The listing builds one solid part. Answer for the finished solid, in the listing's coordinates (mm). Face numbers are marked on the shaded views. A direction names the side the tool comes from. Give positions to 0.01 mm unless a question says otherwise; leave off trailing zeros. Loops run counter-clockwise (first coordinate to the right, second up) from the corner with the lowest first, then second, coordinate; pieces in that order, holes last. Notation, with made-up numbers: (22.25, 72) - (68.25, 72) arc R7 cw to (68.25, 80) - close; hole circle Ø11 at (8.25, -5). An arc over 180 degrees is marked (long way). Answer as CSV lines item,"result". Start each with the question number.
1) A cutting plane is placed at B-B (x = -6.7). Determine the outline of the cut face in (y, z), and give its area (3 significant figures).
2) Flat-ended cylindrical pins translate along their axes: pin 1 (4 mm diameter, centred on x = -8.5, y = 7.5, fed in from +Z); pin 2 (5 mm diameter, centred on y = 15.9, z = 21.21, fed in from -X); pin 3 (11 mm diameter, centred on x = -4.5, y = 33, fed in from +Z). Find the tip coordinate at first contact, or state that the pin passes through.
3) For a pull along X with two mould halves and no side action, classify the marked faces 3, 4 and 5 as pulls with the +X half, pulls with the -X half, needs draft (parallel to the pull), parting line crosses it, or undercut.
4) For the marked faces 1 and 2, determine the directions among +Z, -Z, +X, -X, +Y, -Y from which every point of the face is accessible in a straight line to the end or side of a thin tool.
5) A cutting plane is placed at A-A (x = 18). Determine the outline of the cut face in (y, z).
6) Find the intervals of material crossed by line 1 along Y through (x, z) = (47.55, 3.4); line 2 along X through (y, z) = (53, 36); line 3 along X through (y, z) = (58, 27), in increasing order.
7) A cutting plane is placed at C-C (x = -34). Determine the outline of the cut face in (y, z).
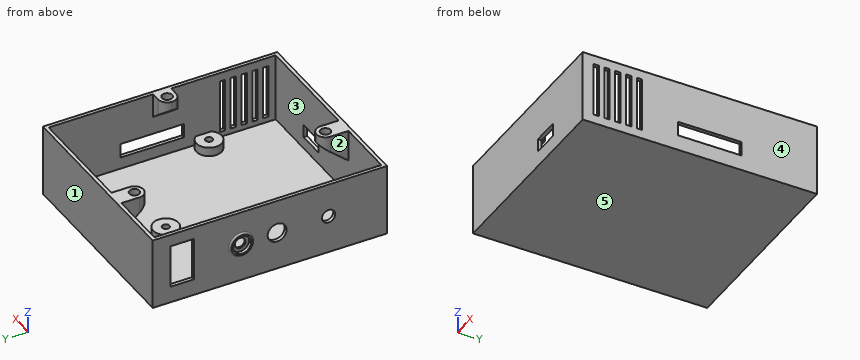
```python
from build123d import *

# Parameters (mm, degrees)
SKETCH1_W                = 110
SKETCH1_H                = 130
BOSS_EXTRUDE1_DEPTH      = 40
SHELL1_T                 = -2
SKETCH2_W                = 15
SKETCH2_H                = 7.298661228
CUT_EXTRUDE1_DEPTH       = 2
SKETCH3_W                = 8
SKETCH3_H                = 35
CUT_EXTRUDE2_DEPTH       = 2
SKETCH5_R                = 3
SKETCH5_R_2              = 5.25
SKETCH5_R_3              = 3.7
SKETCH5_W                = 24
SKETCH5_H                = 13
CUT_EXTRUDE3_DEPTH       = 2
SKETCH6_W                = 30
SKETCH6_H                = 3
CUT_EXTRUDE4_DEPTH       = 2
SKETCH7_R                = 7
SKETCH7_R_2              = 2
BOSS_EXTRUDE2_DEPTH      = 5
BOSS_EXTRUDE3_DEPTH      = 5
FILLET1_R                = 5
BOSS_EXTRUDE4_DEPTH      = 5
BOSS_EXTRUDE4_DEPTH_BACK = 5
FILLET2_R                = 5
CUT_EXTRUDE9_REACH       = 96.074
SKETCH11_R               = 2.8
CUT_EXTRUDE10_REACH      = 96.074
SKETCH13_R               = 2.85
FILLET1_OF_MIRROR1_R     = 5
SKETCH14_R               = 5
CUT_EXTRUDE11_DEPTH      = 1
BOSS_EXTRUDE5_START      = 1
SKETCH15_R               = 6
SKETCH15_R_2             = 5
BOSS_EXTRUDE5_DEPTH      = 1
FILLET3_R                = 1


with BuildPart() as part:
    # Sketch1 → Boss-Extrude1 (new body)
    with BuildSketch(Plane.XY):
        Rectangle(SKETCH1_W, SKETCH1_H)
    extrude(amount=BOSS_EXTRUDE1_DEPTH)

    # Shell1
    shell1_openings = [part.faces().sort_by_distance(p)[0] for p in [
        (0, 0, 40),
    ]]
    offset(amount=SHELL1_T, openings=shell1_openings, kind=Kind.INTERSECTION)

    # Sketch2 → Cut-Extrude1 (cut)
    with BuildSketch(Plane.XZ.offset(65)):
        with Locations((17.5, 12.249330614)):
            Rectangle(SKETCH2_W, SKETCH2_H)
    extrude(amount=-CUT_EXTRUDE1_DEPTH, mode=Mode.SUBTRACT)

    # Sketch3 → Cut-Extrude2 (cut)
    with BuildSketch(Plane(origin=(55, 0, 0), x_dir=(0, 0, -1), z_dir=(1, 0, 0))):
        with Locations((-12.6, 5.5)):
            Rectangle(SKETCH3_W, SKETCH3_H)
    extrude(amount=-CUT_EXTRUDE2_DEPTH, mode=Mode.SUBTRACT)

    # Sketch5 → Cut-Extrude3 (cut)
    with BuildSketch(Plane.ZY.offset(55)):
        with Locations((21.210132709, 15.904045732)):
            Circle(SKETCH5_R)
        with Locations((21.210132709, -4.045954268)):
            Circle(SKETCH5_R_2)
        with Locations((21.210132709, -32.595954268)):
            Circle(SKETCH5_R_3)
        with Locations((21.210132709, 48.5)):
            Rectangle(SKETCH5_W, SKETCH5_H)
    extrude(amount=-CUT_EXTRUDE3_DEPTH, mode=Mode.SUBTRACT)

    # Sketch6 → Cut-Extrude4 (cut)
    with BuildSketch(Plane(origin=(55, 0, 0), x_dir=(0, 0, -1), z_dir=(1, 0, 0))):
        with Locations((-20, -33.5)):
            Rectangle(SKETCH6_W, SKETCH6_H)
        with Locations((-20, -39.5)):
            Rectangle(SKETCH6_W, SKETCH6_H)
        with Locations((-20, -45.5)):
            Rectangle(SKETCH6_W, SKETCH6_H)
        with Locations((-20, -51.5)):
            Rectangle(SKETCH6_W, SKETCH6_H)
        with Locations((-20, -57.5)):
            Rectangle(SKETCH6_W, SKETCH6_H)
    extrude(amount=-CUT_EXTRUDE4_DEPTH, mode=Mode.SUBTRACT)

    # Sketch7 → Boss-Extrude2 (add)
    # profile 1 of 2: a face of its own
    with BuildSketch(Plane.XY.offset(2)):
        with Locations((-6.7, 30.999839281)):
            Circle(SKETCH7_R)
        with Locations((-6.7, 30.999839281)):
            Circle(SKETCH7_R_2, mode=Mode.SUBTRACT)
    # profile 2 of 2: a face of its own
    with BuildSketch(Plane.XY.offset(2)):
        with Locations((47.55, -23.000160719)):
            Circle(SKETCH7_R)
        with Locations((47.55, -23.000160719)):
            Circle(SKETCH7_R_2, mode=Mode.SUBTRACT)
    extrude(amount=BOSS_EXTRUDE2_DEPTH)

    # Sketch9 → Boss-Extrude3 (add, symmetric)
    with BuildSketch(Plane(origin=(-15, 0, 0), x_dir=(0, 0, -1), z_dir=(1, 0, 0))):
        Polygon((-40, 63), (-40, 48), (-35, 48), (-22.413505532, 63), align=None)
    boss_extrude3 = extrude(amount=BOSS_EXTRUDE3_DEPTH, both=True)

    # Fillet1
    fillet1_edges = [part.edges().sort_by_distance(p)[0] for p in [
        (-10, 48, 37.5),
        (-20, 48, 37.5),
    ]]
    fillet(fillet1_edges, radius=FILLET1_R - 0.0001)  # a hair under: the kernel refuses the full size

    # Sketch10 → Boss-Extrude4 (add, two sides: drawn at the far end of the back side and taken through both)
    with BuildSketch(Plane(origin=(0, 0, 0), x_dir=(1, 0, 0), z_dir=(0, 1, 0)).offset(-BOSS_EXTRUDE4_DEPTH_BACK)):
        Polygon((53, -26.609003688), (53, -40), (43, -40), (43, -35), align=None)
    extrude(amount=BOSS_EXTRUDE4_DEPTH + BOSS_EXTRUDE4_DEPTH_BACK)

    # Fillet2
    fillet2_edges = [part.edges().sort_by_distance(p)[0] for p in [
        (43, 5, 37.5),
        (43, -5, 37.5),
    ]]
    fillet(fillet2_edges, radius=FILLET2_R - 0.0001)  # a hair under: the kernel refuses the full size

    # Cut-Extrude9: up to this plane
    cut_extrude9_end = Plane(origin=(-20, 48, 35), z_dir=(0, -0.6427876096865434, -0.7660444431189748))
    # Sketch11 → Cut-Extrude9 (cut, up to the surface)
    with BuildSketch(Plane.XY.offset(40), mode=Mode.PRIVATE) as cut_extrude9_sk1:
        with Locations((-15, 53)):
            Circle(SKETCH11_R)
    cut_extrude9_tool1 = split(extrude(cut_extrude9_sk1.sketch, amount=-CUT_EXTRUDE9_REACH, mode=Mode.PRIVATE), bisect_by=cut_extrude9_end, keep=Keep.BOTH, mode=Mode.PRIVATE)
    cut_extrude9 = cut_extrude9_tool1.solids().sort_by_distance((-15, 53, 40))[0]
    add(cut_extrude9, mode=Mode.SUBTRACT)

    # Cut-Extrude10: up to this plane
    cut_extrude10_end = Plane(origin=(43, -5, 35), z_dir=(-0.6427876096865458, 0, -0.7660444431189727))
    # Sketch13 → Cut-Extrude10 (cut, up to the surface)
    with BuildSketch(Plane.XY.offset(40), mode=Mode.PRIVATE) as cut_extrude10_sk1:
        with Locations((48, 0)):
            Circle(SKETCH13_R)
    cut_extrude10_tool1 = split(extrude(cut_extrude10_sk1.sketch, amount=-CUT_EXTRUDE10_REACH, mode=Mode.PRIVATE), bisect_by=cut_extrude10_end, keep=Keep.BOTH, mode=Mode.PRIVATE)
    add(cut_extrude10_tool1.solids().sort_by_distance((48, 0, 40))[0], mode=Mode.SUBTRACT)

    # Mirror1: Boss-Extrude3, Cut-Extrude9 across plane
    add(boss_extrude3.mirror(Plane.ZX))
    add(cut_extrude9.mirror(Plane.ZX), mode=Mode.SUBTRACT)

    # Fillet1 of Mirror1
    fillet1_of_mirror1_edges = [part.edges().sort_by_distance(p)[0] for p in [
        (-10, -48, 37.5),
        (-20, -48, 37.5),
    ]]
    fillet(fillet1_of_mirror1_edges, radius=FILLET1_OF_MIRROR1_R - 0.0001)  # a hair under: the kernel refuses the full size

    # Sketch14 → Cut-Extrude11 (cut)
    with BuildSketch(Plane.ZY.offset(55)):
        with Locations((21.210132709, 15.904045732)):
            Circle(SKETCH14_R)
    extrude(amount=-CUT_EXTRUDE11_DEPTH, mode=Mode.SUBTRACT)

    # Sketch15 → Boss-Extrude5 (add)
    with BuildSketch(Plane.ZY.offset(55).offset(BOSS_EXTRUDE5_START)):
        with Locations(Location((21.210132709, 15.904045732, 0), (0, 0, 180))):
            Circle(SKETCH15_R)
        with Locations((21.210132709, 15.904045732)):
            Circle(SKETCH15_R_2, mode=Mode.SUBTRACT)
    extrude(amount=-BOSS_EXTRUDE5_DEPTH)

    # Fillet3
    fillet3_edges = [part.edges().sort_by_distance(p)[0] for p in [
        (-55, 15.904045732, 27.210132709),
    ]]
    fillet(fillet3_edges, radius=FILLET3_R - 0.0001)  # a hair under: the kernel refuses the full size


solid = part.part
```
Ans:
1,outline,"(-65, 0) - (65, 0) - (65, 40) - (63, 40) - (63, 2) - (38, 2) - (38, 7) - (33, 7) - (33, 2) - (29, 2) - (29, 7) - (24, 7) - (24, 2) - (-63, 2) - (-63, 40) - (-65, 40) - close"
1,area,"462 mm2"
2,pin 1,"z = 2"
2,pin 2,"x = 53"
2,pin 3,"z = 7"
3,face 3,"undercut"
3,face 4,"pulls with the +X half"
3,face 5,"needs draft"
4,face 1,"+Z, -Z, +X, -X, +Y"
4,face 2,"+Z"
5,outline,"(-65, 0) - (65, 0) - (65, 40) - (63, 40) - (63, 2) - (-63, 2) - (-63, 8.6) - (-65, 8.6) - close; (-65, 15.9) - (-63, 15.9) - (-63, 40) - (-65, 40) - close"
6,line 1,"-65 to -63, -30 to -25, -21 to -16, 63 to 65"
6,line 2,"-55 to -53, -20 to -17.8, -12.2 to -10, 53 to 55"
6,line 3,"-55 to -53, -20 to -10, 53 to 55"
7,outline,"(-65, 0) - (65, 0) - (65, 40) - (63, 40) - (63, 2) - (-63, 2) - (-63, 40) - (-65, 40) - close"
